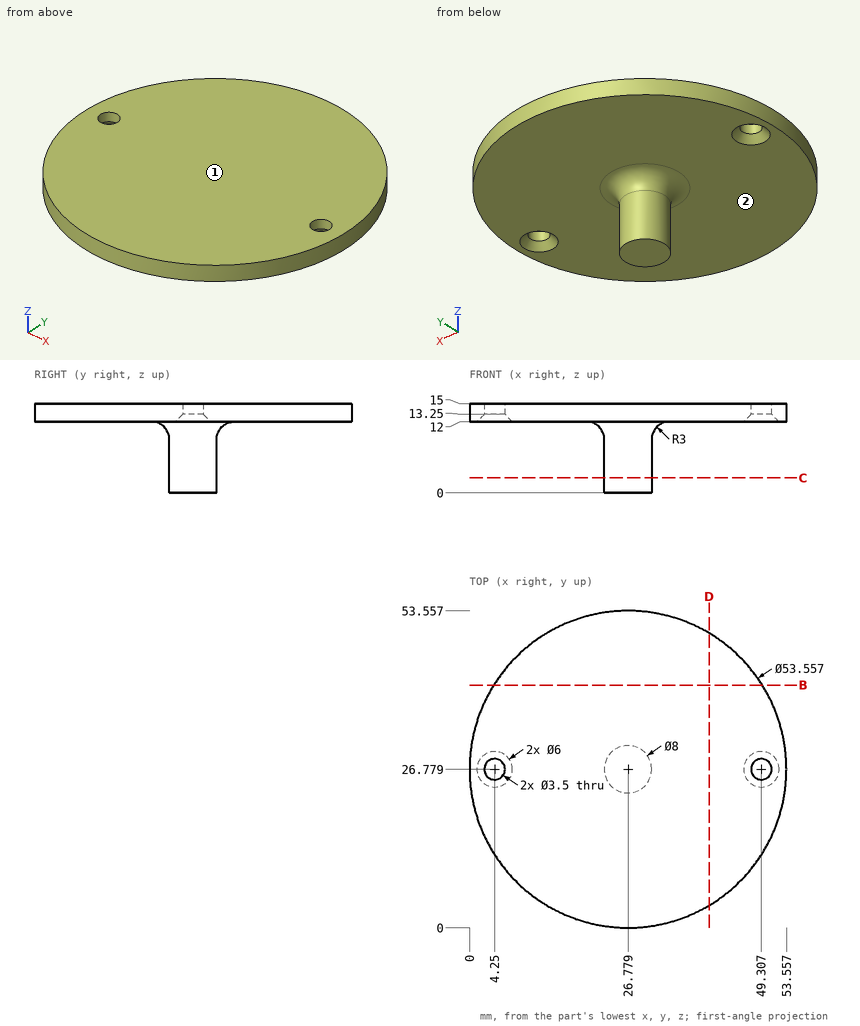
Geometry check sheet. Reference: drawing and pictorial views, mm from the part's lowest x, y, z. A direction names the side the tool comes from. Coordinates: 2 decimals unless noted, no trailing zeros. Loops run counter-clockwise (first coordinate to the right, second up) from the corner with the lowest first, then second, coordinate; pieces in that order, holes last. Notation, with made-up numbers: (22.5, 57.5) - (28.5, 57.5) arc R21 cw to (28.5, 61.5) - close; hole circle Ø5 at (60.25, -38.75). An arc over 180 degrees is marked (long way). Return JSON: item names as keys, results as strings.
1. Section check C-C, the plane z = 2.5. Record the boundary of the cut face in (x, y).
Established:
{"outline": "circle Ø8 at (26.78, 26.78)"}
2. Thickness scan on L1, parallel to Z at x = 43, y = 21.5; L2, parallel to Y at x = 4.25, z = 14.6 (1 decimal); L3, parallel to Y at x = 50, z = 14.25 (1 decimal). Record the ranges inside material, lowest first.
Established:
{"L1": "z = 12 to 15", "L2": "y = 12.3 to 25, 28.5 to 41.3", "L3": "y = 13.4 to 25.2, 28.4 to 40.1"}
3. Go/stop test with flat-tipped pins: pin 1 (2 mm diameter, centred on x = 31, z = 4, fed in from -Y) (1 decimal); pin 2 (8 mm diameter, centred on x = 31, y = 47.5, fed in from -Z); pin 3 (1 mm diameter, centred on y = 28, z = 4.5, fed in from +X). Record where each tip stops, or that it passes through.
Established:
{"pin 1": "stops at y = 24.4", "pin 2": "stops at z = 12", "pin 3": "stops at x = 30.71"}
4. Section check B-B, the plane y = 41. Record the boundary of the cut face in (x, z), then the cut area to 3 significant figures.
Established:
{"outline": "(4.09, 12) - (49.47, 12) - (49.47, 15) - (4.09, 15) - close", "area": "136 mm2"}
5. Tool access check on the marked faces 1 and 2. Record the directions out of +Z, -Z, +X, -X, +Y, -Y that give a thin tool (end or side, any length) a straight path to the whole face; none if there is none.
Established:
{"face 1": "+Z, +X, -X, +Y, -Y", "face 2": "-Z"}
6. Section check D-D, the plane x = 40.5. Record the boundary of the cut face in (y, z) (1 decimal), then the cut area to 3 significant figures.
Established:
{"outline": "(3.8, 12) - (49.8, 12) - (49.8, 15) - (3.8, 15) - close", "area": "138 mm2"}
